```python
from build123d import *

# Parameters (mm, degrees)
F0_R     = 4.5
F0_R_2   = 2.5
F1_DEPTH = 4.25
F0_R_3   = 11
F2_DEPTH = 3.5
F3_SIZE  = 1.5


with BuildPart() as f1:
    # F0 (on Top) → F1 (new body)
    with BuildSketch(Plane.XY):
        Circle(F0_R)
        Circle(F0_R_2, mode=Mode.SUBTRACT)
    extrude(amount=F1_DEPTH)

    # F0 (on Top) → F2 (join)
    with BuildSketch(Plane.XY):
        Circle(F0_R_3)
        Circle(F0_R, mode=Mode.SUBTRACT)
    extrude(amount=F2_DEPTH)

    # F3
    f3_edges = [f1.edges().sort_by_distance(p)[0] for p in [
        (-11, 0, 3.5),
    ]]
    chamfer(f3_edges, length=F3_SIZE)

    # F4: F1 across face


with BuildPart() as f1_1:
    add(f1.part)
    add(f1.part.mirror(Plane(origin=(0, 0, 0), x_dir=(1, 0, 0), z_dir=(0, 0, -1))))


solid = f1_1.part
```
Input: part model. Units: mm. Frame: model coordinates. A direction names the side the tool comes from. Coordinates: 2 decimals unless noted, no trailing zeros. Loops run counter-clockwise (first coordinate to the right, second up) from the corner with the lowest first, then second, coordinate; pieces in that order, holes last. Notation, with made-up numbers: (86, 76.5) - (129, 76.5) arc R13 ccw to (129, 98.5) - close; hole circle Ø11 at (-3, -3). An arc over 180 degrees is marked (long way). Answer in a Markdown table with one row per item.
(1) Cut plane A-A on y = 0. Output: boundary loops of the cut face in (x, z).
Model answer:
| item | result |
|---|---|
| outline | (-11, -2) - (-9.5, -3.5) - (-4.5, -3.5) - (-4.5, -4.25) - (-2.5, -4.25) - (-2.5, 4.25) - (-4.5, 4.25) - (-4.5, 3.5) - (-9.5, 3.5) - (-11, 2) - close; (2.5, -4.25) - (4.5, -4.25) - (4.5, -3.5) - (9.5, -3.5) - (11, -2) - (11, 2) - (9.5, 3.5) - (4.5, 3.5) - (4.5, 4.25) - (2.5, 4.25) - close |
(2) Pin query (flat end, axial travel): P1, Ø4, axis at x = -8, y = 0, coming from the -Z side; P2, Ø9.5, axis at x = -0.5, y = -4.5, coming from the -Z side; P3, Ø1, axis at y = -5, z = -3, coming from the +X side; P4, Ø1, axis at x = 5.5, z = -2.5, coming from the -Y side. Return the tip coordinate at first contact, or that it passes through.
Model answer:
| item | result |
|---|---|
| P1 | stops at z = -3.5 |
| P2 | stops at z = -4.25 |
| P3 | stops at x = 9.29 |
| P4 | stops at y = -9.59 |
(3) Material intervals for L1, parallel to Y at x = 0, z = 1.25; L2, parallel to Y at x = 0, z = -2.25; L3, parallel to Z at x = -5.75, y = -0.5, sorted ascending. Write a range as from..to.
Model answer:
| item | result |
|---|---|
| L1 | y = -11..-2.5, 2.5..11 |
| L2 | y = -10.75..-2.5, 2.5..10.75 |
| L3 | z = -3.5..3.5 |
(4) Cut plane C-C on z = 0.75. Output: boundary loops of the cut face in (x, y), plus the area to 3 significant figures.
Model answer:
| item | result |
|---|---|
| outline | circle Ø22 at (0, 0); hole circle Ø5 at (0, 0) |
| area | 360 mm² |
(5) Mould query, pull axis Y, two halves, no side actions, for faces 4 (the face through (-8, -6, -3)), 5 (the face through (4.1, 2.2, -3.5)), 6 (the face through (-0.54, -2.44, -0.06)). Classes: pulls with the +Y half, pulls with the -Y half, needs draft (parallel to the pull), parting line crosses it, or undercut.
Model answer:
| item | result |
|---|---|
| face 4 | parting line crosses it |
| face 5 | needs draft |
| face 6 | undercut |
(6) Set-up query: faces 1 (the face through (-0.59, 4.46, -3.87)), 2 (the face through (2, -2, -4.25)), 3 (the face through (-0.59, 4.46, 3.87)). Return all of +Z, -Z, +X, -X, +Y, -Y with unobstructed straight access to the full face (end or side cutting, diameter ignored); none if empty.
Model answer:
| item | result |
|---|---|
| face 1 | -Z |
| face 2 | -Z, +X, -X, +Y, -Y |
| face 3 | +Z |
